The figure shows three views and two pictorial views of one solid part (mm, origin at its lowest corner). Answer the questions. Give positions to 0.01 mm unless a question says otherwise; leave off trailing zeros. Write each loop counter-clockwise with the first axis right and the second up, starting at its lowest first coordinate (ties: lowest second). Pieces come first, ordered by that corner, then holes. Notation, with made-up numbers: (30.5, 82.5) -> (49.5, 82.5) arc R16 ccw to (49.5, 99.5) -> close; hole circle Ø3 at (58.25, 87.25). An arc over 180 degrees is marked (long way). Write item = value, one per line. Start each with the question number.
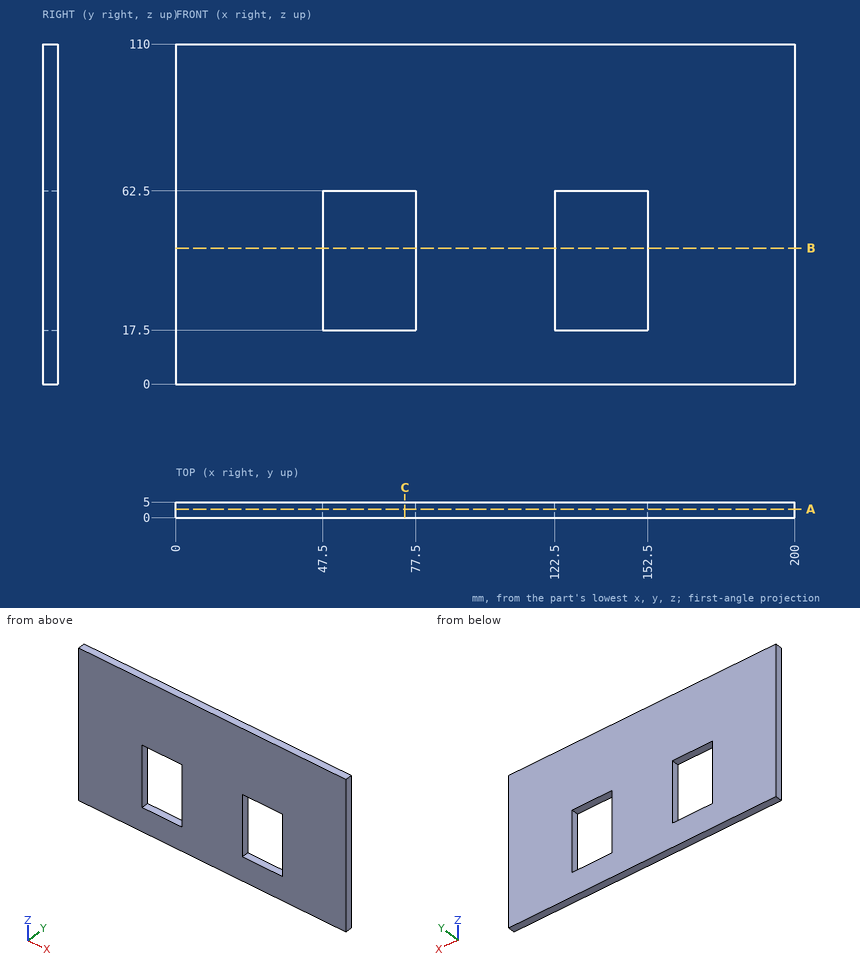
(1) A cutting plane is placed at B-B, the plane z = 44. Write down the section's boundary in (x, y).
(2) Find the intervals of material crossed by line 1 along X through (y, z) = (4.75, 54); line 2 along Z through (x, y) = (123.5, 4.7), in increasing order.
(3) A cutting plane is placed at A-A, the plane y = 2.75. Write down the section's boundary in (x, z).
(4) A cutting plane is placed at C-C, the plane x = 74. Write down the section's boundary in (y, z).
Results list:
q1.outline = (0, 0) -> (47.5, 0) -> (47.5, 5) -> (0, 5) -> close; (77.5, 0) -> (122.5, 0) -> (122.5, 5) -> (77.5, 5) -> close; (152.5, 0) -> (200, 0) -> (200, 5) -> (152.5, 5) -> close
q2.line_1 = 0 to 47.5, 77.5 to 122.5, 152.5 to 200
q2.line_2 = 0 to 17.5, 62.5 to 110
q3.outline = (0, 0) -> (200, 0) -> (200, 110) -> (0, 110) -> close; hole (47.5, 17.5) -> (77.5, 17.5) -> (77.5, 62.5) -> (47.5, 62.5) -> close; hole (122.5, 17.5) -> (152.5, 17.5) -> (152.5, 62.5) -> (122.5, 62.5) -> close
q4.outline = (0, 0) -> (5, 0) -> (5, 17.5) -> (0, 17.5) -> close; (0, 62.5) -> (5, 62.5) -> (5, 110) -> (0, 110) -> close
